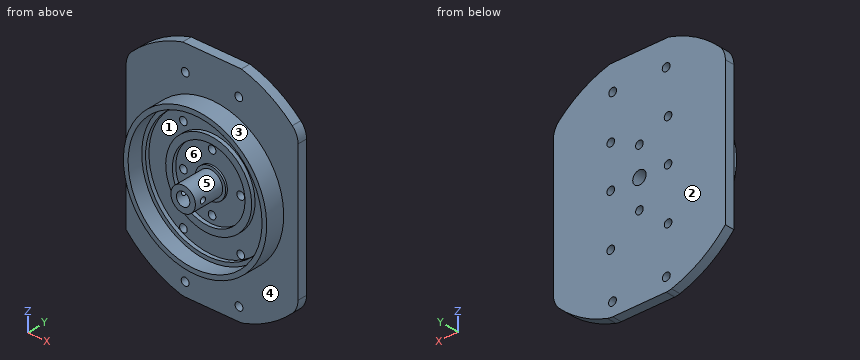
```python
from build123d import *

# Parameters (mm, degrees)
SKETCH2_R                = 6.4
BOSS_EXTRUDE1_DEPTH      = 20
SKETCH3_R                = 8
BOSS_EXTRUDE2_DEPTH      = 1
SKETCH4_R                = 60
BOSS_EXTRUDE3_DEPTH      = 5
SKETCH5_R                = 2
CUT_EXTRUDE1_DEPTH       = 89.746830929
CIRPATTERN1_COUNT        = 4
CUT_EXTRUDE2_DEPTH       = 89.746830929
CUT_EXTRUDE2_DEPTH_BACK  = 89.746830929
SKETCH6_R                = 3.5
CUT_EXTRUDE3_DEPTH       = 89.746830929
CUT_EXTRUDE3_DEPTH_BACK  = 89.746830929
SKETCH7_R                = 2.05
CUT_EXTRUDE4_DEPTH       = 89.746830929
CUT_EXTRUDE6_DEPTH       = 88.407093534
CUT_EXTRUDE6_DEPTH_BACK  = 88.407093534
SKETCH10_R               = 1.5
CUT_EXTRUDE9_DEPTH       = 88.407093563
CUT_EXTRUDE9_DEPTH_BACK  = 4
SKETCH14_R               = 6.4
SKETCH14_R_2             = 3.5
SKETCH16_R               = 37.5
SKETCH16_R_2             = 35.05
BOSS_EXTRUDE4_DEPTH      = 10
SKETCH19_R               = 2
CUT_EXTRUDE10_DEPTH      = 5
SKETCH20_R               = 35.05
SKETCH20_R_2             = 33.05
BOSS_EXTRUDE5_DEPTH      = 2
SKETCH21_R               = 22.5
SKETCH21_R_2             = 19
BOSS_EXTRUDE6_DEPTH      = 2
CUT_EXTRUDE11_DEPTH      = 87.301796067
CUT_EXTRUDE11_DEPTH_BACK = 87.301796067
SKETCH22_OUTSIDE_W       = 155.668
SKETCH22_OUTSIDE_H       = 151.668
SKETCH22_OUTSIDE_W_2     = 90
SKETCH22_OUTSIDE_H_2     = 116
FILLET1_R                = 10


with BuildPart() as part:
    # Sketch2 → Boss-Extrude1 (new body)
    with BuildSketch(Plane(origin=(0, 0, 0), x_dir=(1, 0, 0), z_dir=(0, 1, 0))):
        with Locations(Location((0, 0, 0), (0, 0, 270))):
            Circle(SKETCH2_R)
    extrude(amount=BOSS_EXTRUDE1_DEPTH)

    # Sketch3 → Boss-Extrude2 (add)
    with BuildSketch(Plane(origin=(0, 20, 0), x_dir=(1, 0, 0), z_dir=(0, 1, 0))):
        with Locations(Location((0, 0, 0), (0, 0, 270))):
            Circle(SKETCH3_R)
    extrude(amount=BOSS_EXTRUDE2_DEPTH)

    # Sketch4 → Boss-Extrude3 (add)
    with BuildSketch(Plane(origin=(0, 21, 0), x_dir=(1, 0, 0), z_dir=(0, 1, 0))):
        with Locations(Location((0, 0, 0), (0, 0, 270))):
            Circle(SKETCH4_R)
    extrude(amount=BOSS_EXTRUDE3_DEPTH)

    # Sketch5 → Cut-Extrude1 (cut, symmetric)
    with BuildSketch(Plane(origin=(0, 26, 0), x_dir=(1, 0, 0), z_dir=(0, 1, 0))):
        with Locations(Location((0, 15, 0), (0, 0, 270))):
            Circle(SKETCH5_R)
    cut_extrude1 = extrude(amount=CUT_EXTRUDE1_DEPTH, both=True, mode=Mode.SUBTRACT)

    # CirPattern1: Cut-Extrude1 ×4 about axis
    cirpattern1_axis = Axis((0, 0, 0), (0, 1, 0))
    for i in range(1, CIRPATTERN1_COUNT):
        add(cut_extrude1.rotate(cirpattern1_axis, i * 360 / CIRPATTERN1_COUNT), mode=Mode.SUBTRACT)

    # Sketch6 → Cut-Extrude2 (cut, two sides: drawn at the far end of the back side and taken through both)
    with BuildSketch(Plane(origin=(0, 26, 0), x_dir=(1, 0, 0), z_dir=(0, 1, 0)).offset(-CUT_EXTRUDE2_DEPTH_BACK)):
        with Locations(Location((0, 0, 0), (0, 0, 270))):
            Circle(SKETCH6_R)
    extrude(amount=CUT_EXTRUDE2_DEPTH + CUT_EXTRUDE2_DEPTH_BACK, mode=Mode.SUBTRACT)

    # Sketch7 → Cut-Extrude3 (cut, two sides: drawn at the far end of the back side and taken through both)
    with BuildSketch(Plane(origin=(0, 26, 0), x_dir=(1, 0, 0), z_dir=(0, 1, 0)).offset(-CUT_EXTRUDE3_DEPTH_BACK)):
        with Locations(Location((-14, -44.7, 0), (0, 0, 270))):
            Circle(SKETCH7_R)
        with Locations(Location((14, -44.7, 0), (0, 0, 270))):
            Circle(SKETCH7_R)
        with Locations(Location((-14.1, 51, 0), (0, 0, 270))):
            Circle(SKETCH7_R)
        with Locations(Location((14.1, 51, 0), (0, 0, 270))):
            Circle(SKETCH7_R)
    extrude(amount=CUT_EXTRUDE3_DEPTH + CUT_EXTRUDE3_DEPTH_BACK, mode=Mode.SUBTRACT)

    # Sketch8 → Cut-Extrude4 (cut, symmetric)
    with BuildSketch(Plane(origin=(0, 26, 0), x_dir=(1, 0, 0), z_dir=(0, 1, 0))):
        with BuildLine():
            Line((-15.362291496, 58), (15.362291496, 58))
            ThreePointArc((15.362291496, 58), (0, 60), (-15.362291496, 58))
        make_face()
    cut_extrude4 = extrude(amount=CUT_EXTRUDE4_DEPTH, both=True, mode=Mode.SUBTRACT)

    # Mirror1: Cut-Extrude4 across plane
    add(cut_extrude4.mirror(Plane.XY), mode=Mode.SUBTRACT)

    # Sketch10 → Cut-Extrude6 (cut, two sides: drawn at the far end of the back side and taken through both)
    with BuildSketch(Plane(origin=(0, 0, 0), x_dir=(0, 0, -1), z_dir=(1, 0, 0)).offset(-CUT_EXTRUDE6_DEPTH_BACK)):
        with Locations((0, 8.5)):
            Circle(SKETCH10_R)
    extrude(amount=CUT_EXTRUDE6_DEPTH + CUT_EXTRUDE6_DEPTH_BACK, mode=Mode.SUBTRACT)

    # Sketch14 → Cut-Extrude9 (cut, two sides: drawn at the far end of the back side and taken through both)
    with BuildSketch(Plane.XZ.offset(-CUT_EXTRUDE9_DEPTH_BACK)):
        with Locations(Location((0, 0, 0), (0, 0, 270))):
            Circle(SKETCH14_R)
        with Locations(Location((0, 0, 0), (0, 0, 90))):
            Circle(SKETCH14_R_2, mode=Mode.SUBTRACT)
    extrude(amount=CUT_EXTRUDE9_DEPTH + CUT_EXTRUDE9_DEPTH_BACK, mode=Mode.SUBTRACT)

    # Sketch16 → Boss-Extrude4 (add)
    with BuildSketch(Plane.XZ.offset(-21)):
        with Locations(Location((0, 0, 0), (0, 0, 90))):
            Circle(SKETCH16_R)
        with Locations(Location((0, 0, 0), (0, 0, 270))):
            Circle(SKETCH16_R_2, mode=Mode.SUBTRACT)
    extrude(amount=BOSS_EXTRUDE4_DEPTH)

    # Sketch19 → Cut-Extrude10 (cut)
    with BuildSketch(Plane(origin=(0, 26, 0), x_dir=(1, 0, 0), z_dir=(0, 1, 0))):
        with Locations(Location((-15, 27, 0), (0, 0, 270))):
            Circle(SKETCH19_R)
        with Locations(Location((15, 27, 0), (0, 0, 270))):
            Circle(SKETCH19_R)
        with Locations(Location((15, -22, 0), (0, 0, 270))):
            Circle(SKETCH19_R)
        with Locations(Location((-15, -22, 0), (0, 0, 270))):
            Circle(SKETCH19_R)
    extrude(amount=-CUT_EXTRUDE10_DEPTH, mode=Mode.SUBTRACT)

    # Sketch20 → Boss-Extrude5 (add)
    with BuildSketch(Plane.XZ.offset(-21)):
        with Locations(Location((0, 0, 0), (0, 0, 270))):
            Circle(SKETCH20_R)
        with Locations(Location((0, 0, 0), (0, 0, 270))):
            Circle(SKETCH20_R_2, mode=Mode.SUBTRACT)
    extrude(amount=BOSS_EXTRUDE5_DEPTH)

    # Sketch21 → Boss-Extrude6 (add)
    with BuildSketch(Plane.XZ.offset(-21)):
        with Locations(Location((0, 0, 0), (0, 0, 90))):
            Circle(SKETCH21_R)
        with Locations(Location((0, 0, 0), (0, 0, 270))):
            Circle(SKETCH21_R_2, mode=Mode.SUBTRACT)
    extrude(amount=BOSS_EXTRUDE6_DEPTH)

    # Sketch22 outside → Cut-Extrude11 (cut, two sides: drawn at the far end of the back side and taken through both)
    with BuildSketch(Plane(origin=(0, 26, 0), x_dir=(1, 0, 0), z_dir=(0, 1, 0)).offset(-CUT_EXTRUDE11_DEPTH_BACK)):
        Rectangle(SKETCH22_OUTSIDE_W, SKETCH22_OUTSIDE_H)
        Rectangle(SKETCH22_OUTSIDE_W_2, SKETCH22_OUTSIDE_H_2, mode=Mode.SUBTRACT)
    extrude(amount=CUT_EXTRUDE11_DEPTH + CUT_EXTRUDE11_DEPTH_BACK, mode=Mode.SUBTRACT)

    # Fillet1
    fillet1_edges = [part.edges().sort_by_distance(p)[0] for p in [
        (45, 23.5, 39.686269666),
        (45, 23.5, -39.686269666),
        (-45, 23.5, 39.686269666),
        (-15.362291496, 23.5, -58),
        (15.362291496, 23.5, -58),
    ]]
    fillet(fillet1_edges, radius=FILLET1_R)


solid = part.part
```
Read the model definition and answer for the solid it produces. Units are mm, in the model's axes. Face numbers are marked on the shaded views. A direction names the side the tool comes from. Give positions to 0.01 mm unless a question says otherwise; leave off trailing zeros. Order: outer loops, then holes, each group sorted by start corner. A loop starts at its lowest first (then second) coordinate and runs counter-clockwise, first axis right, second up.
(1) Find section C-C (z = 15). Give the vertices of the cut face in (x, y), plus the area to 3 significant figures.
(2) For a pull along X with two mould halves and no side action, classify the marked faces 3, 4, 5 and 6 as released by +X, released by -X, zero draft, split by the parting line, or undercut.
(3) Find section A-A (y = 15.75). Give the vertices of the cut face in (x, z).
(4) Find section B-B (z = 44.7). Give the vertices of the cut face in (x, y), plus the area to 3 significant figures.
(5) Straight lines are drawn through the part: L1, parallel to X at y = 24.5, z = 22; L2, parallel to X at y = 15, z = 0; L3, parallel to X at y = 13.75, z = 2.5. For each, find the intervals that lie inside material, in ascending order.
(6) Given pin 1 (1.8 mm diameter, centred on y = 8.5, z = 0, fed in from -X); pin 2 (1.5 mm diameter, centred on x = 14, z = 19.5, fed in from -Y); pin 3 (2 mm diameter, centred on y = 17, z = 23.5, fed in from -X); pin 4 (3 mm diameter, centred on x = 12.5, y = 10, fed in from -Z), each flat-ended and moving along its own axis, determine where each tip first touches the part or whether it passes through.
(7) For the marked faces 1 and 2, determine the directions among +Z, -Z, +X, -X, +Y, -Y from which every point of the face is accessible in a straight line to the end or side of a thin tool.
(8) Find section D-D (x = -24.5). Give the vertices of the cut face in (y, z), plus the area to 3 significant figures.
Result sheet:
1. outline: (-45, 21) - (-34.37, 21) - (-34.37, 11) - (-31.68, 11) - (-31.68, 19) - (-29.45, 19) - (-29.45, 21) - (-16.77, 21) - (-16.77, 19) - (-11.66, 19) - (-11.66, 21) - (-2, 21) - (-2, 26) - (-45, 26) - close; (2, 21) - (11.66, 21) - (11.66, 19) - (16.77, 19) - (16.77, 21) - (29.45, 21) - (29.45, 19) - (31.68, 19) - (31.68, 11) - (34.37, 11) - (34.37, 21) - (45, 21) - (45, 26) - (2, 26) - close
1. area: 513 mm2
2. face 3: split by the parting line
2. face 4: zero draft
2. face 5: undercut
2. face 6: undercut
3. outline: circle Ø75 at (0, 0); circle Ø12.8 at (0, 0); hole circle Ø70.1 at (0, 0); hole circle Ø7 at (0, 0)
4. outline: (-40.02, 21) - (-16.05, 21) - (-16.05, 26) - (-40.02, 26) - close; (-11.95, 21) - (11.95, 21) - (11.95, 26) - (-11.95, 26) - close; (16.05, 21) - (40.02, 21) - (40.02, 26) - (16.05, 26) - close
4. area: 359 mm2
5. L1: x = -45 to -17, -13 to 13, 17 to 45
5. L2: x = -37.5 to -35.05, -6.4 to -3.5, 3.5 to 6.4, 35.05 to 37.5
5. L3: x = -37.42 to -34.96, -5.89 to -2.45, 2.45 to 5.89, 34.96 to 37.42
6. pin 1: passes through
6. pin 2: stops at y = 21
6. pin 3: stops at x = -30
6. pin 4: stops at z = -35.73
7. face 1: -Y
7. face 2: +Z, -Z, +X, -X, +Y
8. outline: (11, -28.39) - (21, -28.39) - (21, -54.77) - (26, -54.77) - (26, 54.77) - (21, 54.77) - (21, 28.39) - (11, 28.39) - (11, 25.06) - (19, 25.06) - (19, 22.18) - (21, 22.18) - (21, -22.18) - (19, -22.18) - (19, -25.06) - (11, -25.06) - close
8. area: 626 mm2
